Here's how the part is built. I have some questions about the finished solid (model axes, mm). Give positions to 0.01 mm unless a question says otherwise; leave off trailing zeros. Write each loop counter-clockwise with the first axis right and the second up, starting at its lowest first coordinate (ties: lowest second). Pieces come first, ordered by that corner, then holes. Notation, with made-up numbers: (80, 17.25) - (117, 17.25) arc R22 ccw to (117, 33.25) - close; hole circle Ø3 at (25.25, 53). An arc over 180 degrees is marked (long way). Use a Markdown table: item, result.
```python
from build123d import *

# Parameters (mm, degrees)
PAD006_DEPTH            = 300
PAD007_DEPTH            = 10
PAD010_DEPTH            = 10
POCKET001_DEPTH         = 27.5
PAD016_DEPTH            = 300
CHAMFER007_SIZE         = 0.3
CHAMFER008_SIZE         = 0.3
SKETCH018_W             = 1.5
SKETCH018_H             = 12
POCKET002_DEPTH         = 19.201
SKETCH025_W             = 1
SKETCH025_H             = 11
POCKET005_DEPTH         = 0.5
BODY002_PLACEMENT_ANGLE = 90


with BuildPart() as part:
    # Sketch008 → Pad006 (new body)
    with BuildSketch(Plane.XY):
        Polygon((3.8, 3.1), (3.8, 0), (0, 0), (-7.1, 7.1), (0, 14.2), (3.8, 14.2), (3.8, 11.1), (2.2, 11.1), (2.2, 12.6), (1, 12.6), (1, 1.6), (2.2, 1.6), (2.2, 3.1), align=None)
    extrude(amount=PAD006_DEPTH)

    # Sketch010 → Pad007 (join)
    with BuildSketch(Plane(origin=(0, 0, 0), x_dir=(-1, 0, 0), z_dir=(0, 0, -1))):
        Polygon((-3.8, 14.2), (-5.8, 19.2), (6.2, 19.2), (4.2, 14.2), align=None)
    extrude(amount=-PAD007_DEPTH)

    # Sketch013 → Pad010 (join)
    with BuildSketch(Plane(origin=(0, 0, 0), x_dir=(-1, 0, 0), z_dir=(0, 0, -1))):
        Polygon((4.2, 14.2), (7.1, 7.1), (0, 14.2), align=None)
    extrude(amount=-PAD010_DEPTH)

    # Sketch014 (on DatumPlane) → Pocket001 (cut, symmetric)
    with BuildSketch(Plane.XY.offset(150)):
        Polygon((0, 12.785786), (-5.685786, 7.1), (0, 1.414214), align=None)
    extrude(amount=POCKET001_DEPTH, both=True, mode=Mode.SUBTRACT)

    # Sketch021 → Pad016 (join)
    with BuildSketch(Plane.XY):
        Polygon((3.8, 0), (14.406602, -10.606602), (15.537973, -9.475231), (3.8, 2.262742), align=None)
    extrude(amount=PAD016_DEPTH)

    # Chamfer007
    chamfer007_edges = [part.edges().sort_by_distance(p)[0] for p in [
        (-5.2, 16.7, 0),
        (-5.65, 10.65, 0),
        (-3.55, 3.55, 0),
        (9.103301, -5.303301, 0),
        (9.103301, -5.303301, 300),
        (2.2, 2.35, 0),
        (14.972287, -10.040916, 0),
        (14.972287, -10.040916, 300),
        (1, 7.1, 0),
        (-0.2, 19.2, 0),
        (1.9, 0, 0),
        (1.6, 1.6, 0),
        (1.6, 12.6, 0),
        (2.2, 11.85, 0),
        (1.9, 0, 300),
        (-3.55, 3.55, 300),
        (-3.55, 10.65, 300),
        (1.9, 14.2, 300),
        (2.2, 2.35, 300),
        (1.6, 1.6, 300),
        (1, 7.1, 300),
        (1.6, 12.6, 300),
        (2.2, 11.85, 300),
        (14.406602, -10.606602, 150),
        (15.537973, -9.475231, 150),
        (3, 11.1, 0),
        (3.8, 12.65, 0),
        (4.8, 16.7, 0),
        (9.668986, -3.606245, 0),
        (3.8, 2.681371, 0),
        (3, 3.1, 0),
        (9.668986, -3.606245, 300),
        (3.8, 12.65, 300),
        (3.8, 2.681371, 300),
        (3, 3.1, 300),
        (3, 11.1, 300),
    ]]
    chamfer(chamfer007_edges, length=CHAMFER007_SIZE)

    # Chamfer008
    chamfer008_edges = [part.edges().sort_by_distance(p)[0] for p in [
        (-6.2, 19.2, 5.15),
        (5.8, 19.2, 5.15),
        (-5.65, 10.65, 10),
        (-5.2, 16.7, 10),
        (-0.2, 19.2, 10),
        (4.8, 16.7, 10),
    ]]
    chamfer(chamfer008_edges, length=CHAMFER008_SIZE)

    # Sketch018 (on Face32 of Chamfer008) → Pocket002 (cut, through all)
    with BuildSketch(Plane.XZ):
        with Locations((-3.75, 21)):
            Rectangle(SKETCH018_W, SKETCH018_H)
        Polygon((0, 15), (0, 27), (2.2, 27), (2.2, 15), (2.2, 12.8), align=None)
    extrude(amount=-POCKET002_DEPTH, mode=Mode.SUBTRACT)

    # Sketch025 (on Face57 of Pocket002) → Pocket005 (cut)
    with BuildSketch(Plane(origin=(0, 0, 27), x_dir=(1, 0, 0), z_dir=(0, 0, -1))):
        with Locations((0.5, -7.1)):
            Rectangle(SKETCH025_W, SKETCH025_H)
    extrude(amount=-POCKET005_DEPTH, mode=Mode.SUBTRACT)


with BuildPart() as part_1:
    # Body002 placement: moved
    add(part.part.moved(Location((53, 0.8, 0))).rotate(Axis((53, 0.8, 0), (0, 0, 1)), BODY002_PLACEMENT_ANGLE))


solid = part_1.part
```
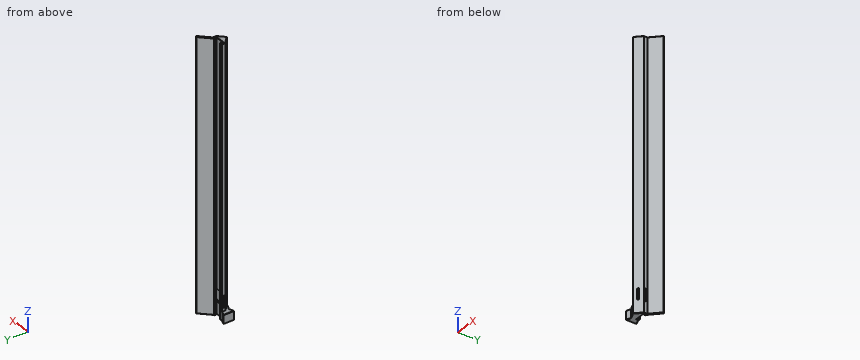
Item 1: If we section it at C-C, the plane x = 56.5: Write out the boundary of the cut face in (y, z), plus the area to 3 significant figures.
Values:
| item | result |
|---|---|
| outline | (8.1, 0.3) - (8.52, 0) - (9.94, 0) - (10.36, 0.3) - (10.36, 299.7) - (9.94, 300) - (8.52, 300) - (8.1, 299.7) - close |
| area | 679 mm2 |
Item 2: If we section it at A-A, the plane z = 154: Write out the boundary of the cut face in (x, y), plus the area to 3 significant figures.
Values:
| item | result |
|---|---|
| outline | (38.8, 0.8) - (45.9, -6.3) - (53, 0.8) - (53, 4.6) - (63.39, 14.99) - (63.39, 15.42) - (62.69, 16.13) - (62.26, 16.13) - (50.74, 4.6) - (49.9, 4.6) - (49.9, 3) - (51.4, 3) - (51.4, 1.8) - (40.4, 1.8) - (40.4, 3) - (41.9, 3) - (41.9, 4.6) - (38.8, 4.6) - close; hole (40.21, 0.8) - (45.9, -4.89) - (51.59, 0.8) - close |
| area | 71.2 mm2 |
Item 3: If we section it at B-B, the plane z = 227.5: Write out the boundary of the cut face in (x, y), plus the area to 3 significant figures.
Values:
| item | result |
|---|---|
| outline | (38.8, 0.8) - (45.9, -6.3) - (53, 0.8) - (53, 4.6) - (63.39, 14.99) - (63.39, 15.42) - (62.69, 16.13) - (62.26, 16.13) - (50.74, 4.6) - (49.9, 4.6) - (49.9, 3) - (51.4, 3) - (51.4, 1.8) - (40.4, 1.8) - (40.4, 3) - (41.9, 3) - (41.9, 4.6) - (38.8, 4.6) - close |
| area | 104 mm2 |
Item 4: Will these pins go through, and if not, where does the flat tip stop? pin 1 Ø1.1 at (y, z) = (2.5, 212) entering from -X; pin 2 Ø12 at (x, z) = (44.5, 8) entering from +Y; pin 3 Ø0.9 at (x, z) = (51, 100.5) entering from -Y.
Values:
| item | result |
|---|---|
| pin 1 | stops at x = 38.8 |
| pin 2 | stops at y = 4.72 |
| pin 3 | stops at y = -1.65 |
Item 5: I need wall thicknesses on line 1 along Z through (x, y) = (44.5, -3.25); line 2 along X through (y, z) = (2, 114); line 3 along X through (y, z) = (-2, 281). Which ranges of each line are inside material? Lowest first, please. Write a range as [from, to].
Values:
| item | result |
|---|---|
| line 1 | z = [0, 15], [27, 122.5], [177.5, 300] |
| line 2 | x = [38.8, 40.4], [51.4, 53] |
| line 3 | x = [41.6, 50.2] |
